The listing builds one solid part. Answer for the finished solid, in the listing's coordinates (mm). Face numbers are marked on the shaded views. A direction names the side the tool comes from. Round coordinates to 2 decimals unless told otherwise and drop trailing zeros. Loops run counter-clockwise (first coordinate to the right, second up) from the corner with the lowest first, then second, coordinate; pieces in that order, holes last. Notation, with made-up numbers: (25.5, -5) - (57.5, -5) arc R33 ccw to (57.5, 31) - close; hole circle Ø11 at (80.5, 58.25). An arc over 180 degrees is marked (long way). One line per item, written item: value.
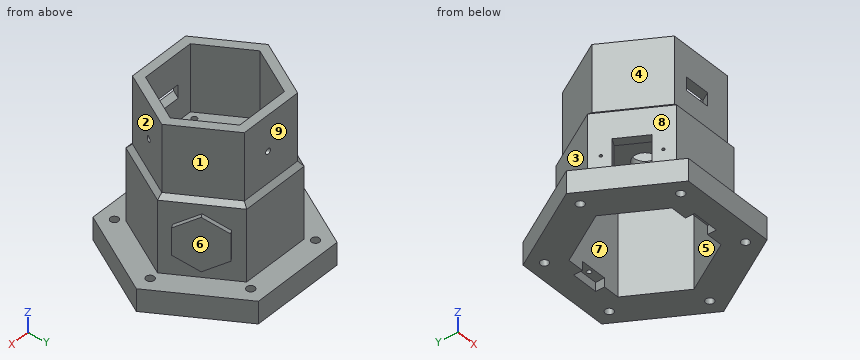
Autodesk Inventor part; units mm, degrees
ref_plane "Work Plane1" through (0, 0, 35) normal (0, 0, -1) x (-1, 0, 0)
ref_plane "Work Plane2" through (-36.2556, -62.7965, 85) normal (-0.5, 0.866, 0) x (0.866, 0.5, 0)
ref_plane "YZ Plane" through (0, 0, 0) normal (1, 0, 0) x (0, 1, 0)
sketch "Sketch1" plane through (0, 0, 0) normal (0, 0, 1) x (1, 0, 0)
  circle A0 centre (0, 0) radius 12.5
  circle A1 centre (51, 0) radius 3
  circle A2 centre (25.5, 44.1673) radius 3
  circle A3 centre (-25.5, 44.1673) radius 3
  circle A4 centre (-51, 0) radius 3
  circle A5 centre (-25.5, -44.1673) radius 3
  circle A6 centre (25.5, -44.1673) radius 3
  line L0 (57.5, 0) -> (28.75, -49.7965)
  line L1 (28.75, -49.7965) -> (-28.75, -49.7965)
  line L2 (-28.75, -49.7965) -> (-57.5, 0)
  line L3 (-57.5, 0) -> (-28.75, 49.7965)
  line L4 (-28.75, 49.7965) -> (28.75, 49.7965)
  line L5 (28.75, 49.7965) -> (57.5, 0)
  line L6 (-30.4821, 52.7965) -> (-60.9641, 0)
  line L7 (-60.9641, 0) -> (-30.4821, -52.7965)
  line L8 (-30.4821, -52.7965) -> (30.4821, -52.7965)
  line L9 (30.4821, -52.7965) -> (60.9641, 0)
  line L10 (60.9641, 0) -> (30.4821, 52.7965)
  line L11 (30.4821, 52.7965) -> (-30.4821, 52.7965)
  dimension "d0" = 25
  dimension "d1" = 6
  dimension "d2" = 51
  dimension "d5" = 360
  dimension "d7" = 115
  dimension "d8" = 3
extrude "Extrusion1" add sketch "Sketch1" along normal blind 10 contours L0 L1 L2 L3 L4 L5 | L11 L10 L9 L8 L7 L6
sketch "Sketch2" plane through (0, 0, 0) normal (0, 0, -1) x (-1, 0, 0)
  circle A0 centre (0, 0) radius 12.5
  circle A1 centre (-25.5, -44.1673) radius 3
  circle A2 centre (25.5, -44.1673) radius 3
  circle A3 centre (51, 0) radius 3
  circle A4 centre (25.5, 44.1673) radius 3
  circle A5 centre (-25.5, 44.1673) radius 3
  circle A6 centre (-51, 0) radius 3
  line L0 (30.4821, 52.7965) -> (60.9641, 0)
  line L1 (-30.4821, 52.7965) -> (30.4821, 52.7965)
  line L2 (-60.9641, 0) -> (-30.4821, 52.7965)
  line L3 (-30.4821, -52.7965) -> (-60.9641, 0)
  line L4 (30.4821, -52.7965) -> (-30.4821, -52.7965)
  line L5 (60.9641, 0) -> (30.4821, -52.7965)
  line L6 (36.2556, -62.7965) -> (-36.2556, -62.7965)
  line L7 (-36.2556, -62.7965) -> (-72.5111, 0)
  line L8 (-72.5111, 0) -> (-36.2556, 62.7965)
  line L9 (-36.2556, 62.7965) -> (36.2556, 62.7965)
  line L10 (36.2556, 62.7965) -> (72.5111, 0)
  line L11 (72.5111, 0) -> (36.2556, -62.7965)
  dimension "d11" = 10
extrude "Extrusion2" add sketch "Sketch2" against normal blind 85 contours L6 L7 L8 L9 L10 L11
ref_plane "Work Plane1" through (0, 0, 35) normal (0, 0, -1) x (-1, 0, 0)
sketch "Sketch4" plane through (0, 0, 35) normal (0, 0, -1) x (-1, 0, 0)
  line L0 (36.2556, -62.7965) -> (-36.2556, -62.7965)
  line L1 (19.7879, -62.7965) -> (14.0144, -52.7965)
  line L2 (30.4821, -52.7965) -> (-30.4821, -52.7965)
  line L3 (-14.8536, -52.7965) -> (14.0144, -52.7965)
  line L4 (-14.8536, -52.7965) -> (-9.0801, -62.7965)
  line L5 (-9.0801, -62.7965) -> (19.7879, -62.7965)
  point P0 (0, 0)
  point P1 (11.6009, -5.3708)
  dimension "d28" = 60
  dimension "d29" = 28.868
  dimension "d30" = 21.402
extrude "Extrusion4" cut sketch "Sketch4" against normal blind 15
ref_plane "Work Plane2" through (-36.2556, -62.7965, 85) normal (-0.5, 0.866, 0) x (0.866, 0.5, 0)
sketch "Sketch5" plane through (-36.2556, -62.7965, 85) normal (-0.5, 0.866, 0) x (0.866, 0.5, 0)
  line L0 (125.5929, 85) -> (125.5929, 0)
  circle A0 centre (97.5929, 40) radius 3
  line L1 (115.5929, 75) -> (62.7965, 75)
  point P0 (0, 0)
  dimension "d38" = 6
  dimension "d39" = 35
  dimension "d40" = 28
extrude "Extrusion5" cut sketch "Sketch5" along normal through all both and the other way through all
sketch "Sketch7" plane through (0, 0, 0) normal (0, 0, -1) x (-1, 0, 0)
  line L0 (36.2556, -62.7965) -> (-36.2556, -62.7965)
  line L1 (72.5111, 0) -> (36.2556, -62.7965)
  line L2 (36.2556, 62.7965) -> (72.5111, 0)
  line L3 (-36.2556, 62.7965) -> (36.2556, 62.7965)
  line L4 (-72.5111, 0) -> (-36.2556, 62.7965)
  line L5 (-36.2556, -62.7965) -> (-72.5111, 0) construction
  circle A0 centre (0, 0) radius 12.5
  circle A1 centre (-25.5, -44.1673) radius 3
  circle A2 centre (25.5, -44.1673) radius 3
  circle A3 centre (51, 0) radius 3
  circle A4 centre (25.5, 44.1673) radius 3
  circle A5 centre (-25.5, 44.1673) radius 3
  circle A6 centre (-51, 0) radius 3
  line L6 (-60.9641, 0) -> (-30.4821, 52.7965)
  line L7 (-30.4821, -52.7965) -> (-60.9641, 0) construction
  line L8 (30.4821, -52.7965) -> (-30.4821, -52.7965)
  line L9 (60.9641, 0) -> (30.4821, -52.7965)
  line L10 (30.4821, 52.7965) -> (60.9641, 0)
  line L11 (-30.4821, 52.7965) -> (30.4821, 52.7965)
  line L12 (-78.2846, 0) -> (-39.1423, 67.7965)
  line L13 (-39.1423, 67.7965) -> (39.1423, 67.7965)
  line L14 (39.1423, 67.7965) -> (78.2846, 0)
  line L15 (78.2846, 0) -> (39.1423, -67.7965)
  line L16 (39.1423, -67.7965) -> (-39.1423, -67.7965)
  line L17 (-39.1423, -67.7965) -> (-78.2846, 0)
  line L18 (-33.3688, 57.7965) -> (-66.7376, 0)
  line L19 (-66.7376, 0) -> (-33.3688, -57.7965)
  line L20 (-33.3688, -57.7965) -> (33.3688, -57.7965)
  line L21 (33.3688, -57.7965) -> (66.7376, 0)
  line L22 (66.7376, 0) -> (33.3688, 57.7965)
  line L23 (33.3688, 57.7965) -> (-33.3688, 57.7965)
  dimension "d41" = 5
  dimension "d42" = 5
extrude "Extrusion6" add sketch "Sketch7" along normal blind 100 and the other way blind 10 contours L12 L13 L14 L15 L16 L17
sketch "Sketch8" plane through (0, 0, -100) normal (0, 0, -1) x (-1, 0, 0)
  circle A0 centre (-88.2846, 0) radius 4.5
  circle A1 centre (-44.1423, -76.4567) radius 4.5
  circle A2 centre (44.1423, -76.4567) radius 4.5
  circle A3 centre (88.2846, 0) radius 4.5
  circle A4 centre (44.1423, 76.4567) radius 4.5
  circle A5 centre (-44.1423, 76.4567) radius 4.5
  line L0 (-33.3688, 57.7965) -> (33.3688, 57.7965) construction
  line L1 (33.3688, 57.7965) -> (66.7376, 0) construction
  line L2 (66.7376, 0) -> (33.3688, -57.7965) construction
  line L3 (33.3688, -57.7965) -> (-33.3688, -57.7965) construction
  line L4 (-33.3688, -57.7965) -> (-66.7376, 0) construction
  line L5 (-66.7376, 0) -> (-33.3688, 57.7965) construction
  line L6 (-39.1423, 67.7965) -> (-78.2846, 0)
  line L7 (-78.2846, 0) -> (-39.1423, -67.7965)
  line L8 (-39.1423, -67.7965) -> (39.1423, -67.7965)
  line L9 (39.1423, -67.7965) -> (78.2846, 0)
  line L10 (78.2846, 0) -> (39.1423, 67.7965)
  line L11 (39.1423, 67.7965) -> (-39.1423, 67.7965)
  line L12 (-53.5761, -92.7965) -> (-107.1521, 0)
  line L13 (-107.1521, 0) -> (-53.5761, 92.7965)
  line L14 (-53.5761, 92.7965) -> (53.5761, 92.7965)
  line L15 (53.5761, 92.7965) -> (107.1521, 0)
  line L16 (107.1521, 0) -> (53.5761, -92.7965)
  line L17 (53.5761, -92.7965) -> (-53.5761, -92.7965)
  point P0 (0, 0)
  dimension "d47" = 9
  dimension "d48" = 10
  dimension "d51" = 360
  dimension "d53" = 25
extrude "Extrusion7" add sketch "Sketch8" against normal blind 25
sketch "Sketch9" plane through (0, 0, -100) normal (0, 0, -1) x (-1, 0, 0)
  line L0 (33.3688, -57.7965) -> (-33.3688, -57.7965)
  line L1 (-15, -57.7965) -> (15, -57.7965)
  line L2 (15, -57.7965) -> (15, -67.7965)
  line L3 (15, -67.7965) -> (-15, -67.7965)
  line L4 (-15, -67.7965) -> (-15, -57.7965)
  line L5 (33.3688, 57.7965) -> (-33.3688, 57.7965)
  line L6 (-15, 57.7965) -> (15, 57.7965)
  line L7 (15, 57.7965) -> (15, 67.7965)
  line L8 (15, 67.7965) -> (-15, 67.7965)
  line L9 (-15, 67.7965) -> (-15, 57.7965)
  line L10 (-33.3688, 57.7965) -> (33.3688, 57.7965)
  point P0 (0, 0)
  point P1 (0, 57.7965)
  point P2 (0, -57.7965)
  point P3 (0, 57.7965)
  point P4 (0, 57.7965)
  dimension "d56" = 10
  dimension "d57" = 10
  dimension "d58" = 30
extrude "Extrusion8" cut sketch "Sketch9" against normal blind 10
chamfer "Chamfer1" distance 5 angle 45 6 edges at (-58.7135, 33.8982, 10) (0, 67.7965, 10) (58.7135, 33.8982, 10) (58.7135, -33.8982, 10) (0, -67.7965, 10) (-58.7135, -33.8982, 10)
sketch "Sketch10" plane through (0, 0, -90) normal (0, 0, -1) x (-1, 0, 0)
  line L0 (15, 57.7965) -> (-15, 57.7965) construction
  line L1 (15, 67.7965) -> (15, 57.7965) construction
  line L2 (-15, 67.7965) -> (15, 67.7965) construction
  line L3 (-15, 57.7965) -> (-15, 67.7965) construction
  line L4 (-15, -57.7965) -> (15, -57.7965) construction
  line L5 (-15, -67.7965) -> (-15, -57.7965) construction
  line L6 (15, -67.7965) -> (-15, -67.7965) construction
  line L7 (15, -57.7965) -> (15, -67.7965) construction
  circle A0 centre (0, 62.7965) radius 2.5
  circle A1 centre (0, -62.7965) radius 2.5
  point P0 (0, 0)
  point P1 (0, 67.7965)
  point P2 (0, -57.7965)
  point P3 (-15, 62.7965)
  point P4 (-15, -62.7965)
  dimension "d64" = 5
  dimension "d65" = 5
extrude "Extrusion9" cut sketch "Sketch10" against normal blind 50
sketch "Sketch11" plane through (-78.2846, 0, -75) normal (-0.866, -0.5, 0) x (0, 0, 1)
  line L0 (80, 0) -> (80, -78.2846)
  line L1 (0, 0) -> (80, 0)
  line L2 (0, 0) -> (0, -78.2846)
  line L3 (0, -78.2846) -> (80, -78.2846)
  line L4 (50, -21.6423) -> (15, -21.6423)
  line L5 (15, -21.6423) -> (15, -56.6423)
  line L6 (15, -56.6423) -> (50, -56.6423)
  line L7 (50, -56.6423) -> (50, -21.6423)
  circle A0 centre (32.5, -11.6423) radius 1.5
  circle A1 centre (32.5, -66.6423) radius 1.5
  point P0 (75, -39.1423)
  point P1 (50, -39.1423)
  point P2 (80, -39.1423)
  point P3 (32.5, -21.6423)
  point P4 (32.5, -56.6423)
  dimension "d68" = 35
  dimension "d69" = 35
  dimension "d70" = 15
  dimension "d77" = 3
  dimension "d78" = 3
  dimension "d79" = 10
  dimension "d80" = 10
extrude "Extrusion10" cut sketch "Sketch11" against normal blind 25 contours L7 L6 L5 L4 | A0 | A1
sketch "Sketch12" plane through (78.2846, 0, 5) normal (0.866, 0.5, 0) x (0, 0, -1)
  line L0 (10, 39.1423) -> (25, 65.1231)
  line L1 (25, 65.1231) -> (55, 65.1231)
  line L2 (55, 65.1231) -> (70, 39.1423)
  line L3 (70, 39.1423) -> (55, 13.1615)
  line L4 (55, 13.1615) -> (25, 13.1615)
  line L5 (25, 13.1615) -> (10, 39.1423)
  line L6 (0, 0) -> (0, 78.2846)
  line L7 (80, -14.4338) -> (80, 92.7184)
  point P0 (5, 39.1423)
  point P1 (40, 39.1423)
  point P2 (0, 39.1423)
  dimension "d73" = 60
  dimension "d74" = 40
extrude "Extrusion11" add sketch "Sketch12" along normal blind 5
equation "\"d57\" = d56"
properties part number "TARM15" material "ABS Plastic"
1) A cutting plane is placed at C-C on x = -87. Give the vertices of the cut face in (y, z), and give its area (3 significant figures).
Final values:
outline: (-34.9, -100) - (-4.31, -100) - (-4.31, -75) - (-34.9, -75) - close; (4.31, -100) - (34.9, -100) - (34.9, -75) - (4.31, -75) - close
area: 1,530 mm2
2) Each of these flat-tipped pins is pushed along its axis until it touches: pin 1 Ø6 at (x, z) = (60.5, -76) entering from +Y; pin 2 Ø2 at (x, z) = (41.5, 32) entering from +Y; pin 3 Ø5 at (y, z) = (-62, -94) entering from -X; pin 4 Ø11.5 at (x, y) = (-88.28, 0) entering from -Z. Where does it stop, or does it pass through?
Final values:
pin 1: y = 86
pin 2: y = 55.44
pin 3: x = -72.8
pin 4: z = -100
3) A cutting plane is placed at B-B on z = 14. Give the vertices of the cut face in (x, y).
Final values:
outline: (-72.51, 0) - (-36.26, -62.8) - (36.26, -62.8) - (72.51, 0) - (36.26, 62.8) - (-36.26, 62.8) - close; hole (-60.96, 0) - (-30.48, -52.8) - (30.48, -52.8) - (60.96, 0) - (30.48, 52.8) - (-30.48, 52.8) - close
4) A cutting plane is placed at A-A on x = -25.5. Give the number of separate pieces and of enclosed holes in the cut face, and give its area (3 significant figures).
Final values:
separate pieces: 3
enclosed holes: 0
area: 5,960 mm2
5) Consider L1, parallel to Y at x = 10, z = 20.5; L2, parallel to Y at x = -25.5, z = 4.25; L3, parallel to Y at x = 0, z = -79. Determine where each line is inside the solid, lowest interval first.
Final values:
L1: -62.8 to -52.8, 52.8 to 62.8
L2: -67.8 to -47.17, -41.17 to 41.17, 47.17 to 67.8
L3: -92.8 to -65.3, -60.3 to -57.8, 57.8 to 60.3, 65.3 to 92.8
6) For the marked faces 1, 2, 3, 4 and 5, determine the directions among +Z, -Z, +X, -X, +Y, -Y from which every point of the face is accessible in a straight line to the end or side of a thin tool.
Final values:
face 1: +Z, +X, +Y
face 2: +Z, +X, -Y
face 3: +Z, -X, +Y
face 4: +Z, -X, -Y
face 5: -Z
7) For a pull along X with two mould halves and no side action, classify the marked faces 6, 7, 8 and 9 as released by +X, released by -X, zero draft, split by the parting line, or undercut.
Final values:
face 6: released by +X
face 7: undercut
face 8: released by -X
face 9: zero draft
